Build history of the part. All positions in model axes, mm. A direction names the side the tool comes from. Round coordinates to 2 decimals unless told otherwise and drop trailing zeros. Write each loop counter-clockwise with the first axis right and the second up, starting at its lowest first coordinate (ties: lowest second). Pieces come first, ordered by that corner, then holes. Notation, with made-up numbers: M 61.5,-22 L 114.5,-22 A18 cw 114.5,5 Z; hole C 52,54.25 d9. An arc over 180 degrees is marked long. Use a Markdown table: item, result.
from build123d import *

# Parameters (mm, degrees)
TOP_ENVELOPE_START         = 8
CASEENVELOPE_W             = 92
CASEENVELOPE_H             = 63
TOP_ENVELOPE_DEPTH         = 17
OUTSIDE_R3_R               = 3
SHELL_1_T                  = -2
SIDEPORT_CLEARANCE_1_START = 6.45
SIDEPORT_PROFILE_1_W       = 10.1
SIDEPORT_PROFILE_1_H       = 13
SIDEPORT_CLEARANCE_1_DEPTH = 4.5
SIDEPORT_CLEARANCE_2_START = 6.45
SIDEPORT_PROFILE_2_W       = 7.7
SIDEPORT_PROFILE_2_H       = 13
SIDEPORT_CLEARANCE_2_DEPTH = 4.7
SIDEPORT_CLEARANCE_3_START = 6.45
SIDEPORT_PROFILE_3_W       = 7.7
SIDEPORT_PROFILE_3_H       = 13
SIDEPORT_CLEARANCE_3_DEPTH = 4.7
ENDPORT_CLEARANCE_1_START  = 6.45
ENDPORT_PROFILE_1_W        = 11
ENDPORT_PROFILE_1_H        = 17.3
ENDPORT_CLEARANCE_1_DEPTH  = 14.6
ENDPORT_CLEARANCE_2_START  = 6.45
ENDPORT_PROFILE_2_W        = 11
ENDPORT_PROFILE_2_H        = 14.7
ENDPORT_CLEARANCE_2_DEPTH  = 16.3
ENDPORT_CLEARANCE_3_START  = 6.45
ENDPORT_PROFILE_3_W        = 11
ENDPORT_PROFILE_3_H        = 14.7
ENDPORT_CLEARANCE_3_DEPTH  = 16.3
COOLING_SLOTS_START        = 22.5
COOLING_SLOTS_DEPTH        = 3


with BuildPart() as part:
    # CaseEnvelope → Top_Envelope (new body)
    with BuildSketch(Plane.XY.offset(TOP_ENVELOPE_START)):
        Rectangle(CASEENVELOPE_W, CASEENVELOPE_H)
    extrude(amount=TOP_ENVELOPE_DEPTH)

    # Outside_R3
    outside_r3_edges = [part.edges().sort_by_distance(p)[0] for p in [
        (46, -31.5, 16.5),
        (-46, -31.5, 16.5),
        (-46, 31.5, 16.5),
        (46, 31.5, 16.5),
    ]]
    fillet(outside_r3_edges, radius=OUTSIDE_R3_R)

    # Shell 1
    shell_1_openings = [part.faces().sort_by_distance(p)[0] for p in [
        (0, 0, 8),
    ]]
    offset(amount=SHELL_1_T, openings=shell_1_openings, kind=Kind.INTERSECTION)

    # SidePort_Profile_1 → SidePort_Clearance_1 (cut)
    with BuildSketch(Plane.XY.offset(SIDEPORT_CLEARANCE_1_START)):
        with Locations((-31.3, -33.5)):
            Rectangle(SIDEPORT_PROFILE_1_W, SIDEPORT_PROFILE_1_H)
    extrude(amount=SIDEPORT_CLEARANCE_1_DEPTH, mode=Mode.SUBTRACT)

    # SidePort_Profile_2 → SidePort_Clearance_2 (cut)
    with BuildSketch(Plane.XY.offset(SIDEPORT_CLEARANCE_2_START)):
        with Locations((-16.7, -33.5)):
            Rectangle(SIDEPORT_PROFILE_2_W, SIDEPORT_PROFILE_2_H)
    extrude(amount=SIDEPORT_CLEARANCE_2_DEPTH, mode=Mode.SUBTRACT)

    # SidePort_Profile_3 → SidePort_Clearance_3 (cut)
    with BuildSketch(Plane.XY.offset(SIDEPORT_CLEARANCE_3_START)):
        with Locations((-3.3, -33.5)):
            Rectangle(SIDEPORT_PROFILE_3_W, SIDEPORT_PROFILE_3_H)
    extrude(amount=SIDEPORT_CLEARANCE_3_DEPTH, mode=Mode.SUBTRACT)

    # EndPort_Profile_1 → EndPort_Clearance_1 (cut)
    with BuildSketch(Plane.XY.offset(ENDPORT_CLEARANCE_1_START)):
        with Locations((47.5, -17.8)):
            Rectangle(ENDPORT_PROFILE_1_W, ENDPORT_PROFILE_1_H)
    extrude(amount=ENDPORT_CLEARANCE_1_DEPTH, mode=Mode.SUBTRACT)

    # EndPort_Profile_2 → EndPort_Clearance_2 (cut)
    with BuildSketch(Plane.XY.offset(ENDPORT_CLEARANCE_2_START)):
        with Locations((47.5, 1.1)):
            Rectangle(ENDPORT_PROFILE_2_W, ENDPORT_PROFILE_2_H)
    extrude(amount=ENDPORT_CLEARANCE_2_DEPTH, mode=Mode.SUBTRACT)

    # EndPort_Profile_3 → EndPort_Clearance_3 (cut)
    with BuildSketch(Plane.XY.offset(ENDPORT_CLEARANCE_3_START)):
        with Locations((47.5, 19)):
            Rectangle(ENDPORT_PROFILE_3_W, ENDPORT_PROFILE_3_H)
    extrude(amount=ENDPORT_CLEARANCE_3_DEPTH, mode=Mode.SUBTRACT)

    # Cooling_Slot_Profiles → Cooling_Slots (cut)
    with BuildSketch(Plane.XY.offset(COOLING_SLOTS_START)):
        with BuildLine():
            Line((-23.81, -17.4), (18.81, -17.4))
            ThreePointArc((18.81, -17.4), (19.65145707, -17.05145707), (20, -16.21))
            Line((20, -16.21), (20, -16.19))
            ThreePointArc((20, -16.19), (19.65145707, -15.34854293), (18.81, -15))
            Line((18.81, -15), (-23.81, -15))
            ThreePointArc((-23.81, -15), (-24.65145707, -15.34854293), (-25, -16.19))
            Line((-25, -16.19), (-25, -16.21))
            ThreePointArc((-25, -16.21), (-24.65145707, -17.05145707), (-23.81, -17.4))
        make_face()
        with BuildLine():
            Line((-23.81, -12), (18.81, -12))
            ThreePointArc((18.81, -12), (19.65145707, -11.65145707), (20, -10.81))
            Line((20, -10.81), (20, -10.79))
            ThreePointArc((20, -10.79), (19.65145707, -9.94854293), (18.81, -9.6))
            Line((18.81, -9.6), (-23.81, -9.6))
            ThreePointArc((-23.81, -9.6), (-24.65145707, -9.94854293), (-25, -10.79))
            Line((-25, -10.79), (-25, -10.81))
            ThreePointArc((-25, -10.81), (-24.65145707, -11.65145707), (-23.81, -12))
        make_face()
        with BuildLine():
            Line((-23.81, -6.6), (18.81, -6.6))
            ThreePointArc((18.81, -6.6), (19.65145707, -6.25145707), (20, -5.41))
            Line((20, -5.41), (20, -5.39))
            ThreePointArc((20, -5.39), (19.65145707, -4.54854293), (18.81, -4.2))
            Line((18.81, -4.2), (-23.81, -4.2))
            ThreePointArc((-23.81, -4.2), (-24.65145707, -4.54854293), (-25, -5.39))
            Line((-25, -5.39), (-25, -5.41))
            ThreePointArc((-25, -5.41), (-24.65145707, -6.25145707), (-23.81, -6.6))
        make_face()
        with BuildLine():
            Line((-23.81, -1.2), (18.81, -1.2))
            ThreePointArc((18.81, -1.2), (19.65145707, -0.85145707), (20, -0.01))
            Line((20, -0.01), (20, 0.01))
            ThreePointArc((20, 0.01), (19.65145707, 0.85145707), (18.81, 1.2))
            Line((18.81, 1.2), (-23.81, 1.2))
            ThreePointArc((-23.81, 1.2), (-24.65145707, 0.85145707), (-25, 0.01))
            Line((-25, 0.01), (-25, -0.01))
            ThreePointArc((-25, -0.01), (-24.65145707, -0.85145707), (-23.81, -1.2))
        make_face()
        with BuildLine():
            Line((-23.81, 4.2), (18.81, 4.2))
            ThreePointArc((18.81, 4.2), (19.65145707, 4.54854293), (20, 5.39))
            Line((20, 5.39), (20, 5.41))
            ThreePointArc((20, 5.41), (19.65145707, 6.25145707), (18.81, 6.6))
            Line((18.81, 6.6), (-23.81, 6.6))
            ThreePointArc((-23.81, 6.6), (-24.65145707, 6.25145707), (-25, 5.41))
            Line((-25, 5.41), (-25, 5.39))
            ThreePointArc((-25, 5.39), (-24.65145707, 4.54854293), (-23.81, 4.2))
        make_face()
        with BuildLine():
            Line((-23.81, 9.6), (18.81, 9.6))
            ThreePointArc((18.81, 9.6), (19.65145707, 9.94854293), (20, 10.79))
            Line((20, 10.79), (20, 10.81))
            ThreePointArc((20, 10.81), (19.65145707, 11.65145707), (18.81, 12))
            Line((18.81, 12), (-23.81, 12))
            ThreePointArc((-23.81, 12), (-24.65145707, 11.65145707), (-25, 10.81))
            Line((-25, 10.81), (-25, 10.79))
            ThreePointArc((-25, 10.79), (-24.65145707, 9.94854293), (-23.81, 9.6))
        make_face()
        with BuildLine():
            Line((-23.81, 15), (18.81, 15))
            ThreePointArc((18.81, 15), (19.65145707, 15.34854293), (20, 16.19))
            Line((20, 16.19), (20, 16.21))
            ThreePointArc((20, 16.21), (19.65145707, 17.05145707), (18.81, 17.4))
            Line((18.81, 17.4), (-23.81, 17.4))
            ThreePointArc((-23.81, 17.4), (-24.65145707, 17.05145707), (-25, 16.21))
            Line((-25, 16.21), (-25, 16.19))
            ThreePointArc((-25, 16.19), (-24.65145707, 15.34854293), (-23.81, 15))
        make_face()
    extrude(amount=COOLING_SLOTS_DEPTH, mode=Mode.SUBTRACT)


solid = part.part
Q1. Drop flat-ended pins along their axis: P1, Ø1.6, axis at y = -30.5, z = 9, coming from the -X side; P2, Ø1.6, axis at x = -16, y = -30.5, coming from the -Z side; P3, Ø1, axis at y = -30, z = 9, coming from the +X side. Give the stop position or say it passes through.
Response values:
| item | result |
|---|---|
| P1 | stops at x = -45.75 |
| P2 | stops at z = 11.15 |
| P3 | stops at x = 45.83 |
Q2. Cut at A-A on z = 18.25. Give the cut face in (x, y), and give its area (3 significant figures).
Response values:
| item | result |
|---|---|
| outline | M -46,-28.5 A3 ccw -43,-31.5 L 43,-31.5 A3 ccw 46,-28.5 L 46,-26.45 L 44,-26.45 L 44,-28.5 A1 cw 43,-29.5 L -43,-29.5 A1 cw -44,-28.5 L -44,28.5 A1 cw -43,29.5 L 43,29.5 A1 cw 44,28.5 L 44,26.35 L 46,26.35 L 46,28.5 A3 ccw 43,31.5 L -43,31.5 A3 ccw -46,28.5 Z; M 44,-9.15 L 46,-9.15 L 46,-6.25 L 44,-6.25 Z; M 44,8.45 L 46,8.45 L 46,11.65 L 44,11.65 Z |
| area | 504 mm2 |
Q3. Cut at B-B on y = -13.5. Give the cut face in (x, z).
Response values:
| item | result |
|---|---|
| outline | M -46,8 L -44,8 L -44,23 L 44,23 L 44,21.05 L 46,21.05 L 46,25 L -46,25 Z |
Q4. Which spindle directions (+Z, -Z, +X, -X, +Y, -Y) get a long thin tool onto all of the face, cutting with end or side? Do faces 1 (the flat face through (-3, -1.2, 24)), 2 (the flat face through (-36.35, -31, 9)), 3 (the flat face through (45, 19, 22.75)), 4 (the cylindrical face through (45.1, -30.64, 16.62)), 5 (the flat face through (-1, 31.5, 16)). Say none if no direction does.
Response values:
| item | result |
|---|---|
| face 1 | +Z, -Z |
| face 2 | -Z, -Y |
| face 3 | -Z, +X |
| face 4 | +Z, -Z, +X, -Y |
| face 5 | +Z, -Z, +X, -X, +Y |
Q5. Two-plate mould, pull along Y, no slides. Class faces 6 (the flat face through (-2, -15, 24)), 7 (the cylindrical face through (-45.14, 30.6, 16.62)), 8 (the flat face through (45, 8.45, 15)), 9 (the flat face through (-7.15, -31, 10)): +Y half, -Y half, draft (parallel to the pull), parting line (faces both ways), or undercut.
Response values:
| item | result |
|---|---|
| face 6 | undercut |
| face 7 | +Y half |
| face 8 | undercut |
| face 9 | draft |
Q6. Drill centre lines: L1, parallel to Y at x = -29, z = 14; L2, parallel to X at y = 28.5, z = 19.75; L3, parallel to Z at x = 23, y = 0. Where is each one in solid material? Low to high.
Response values:
| item | result |
|---|---|
| L1 | y = -31.5 to -29.5, 29.5 to 31.5 |
| L2 | x = -46 to -44, 44 to 46 |
| L3 | z = 23 to 25 |
Q7. Cut at C-C on x = -17. Count the separate pieces of the cut face and the enclosed holes in it, and give its area (3 significant figures).
Response values:
| item | result |
|---|---|
| separate pieces | 8 |
| enclosed holes | 0 |
| area | 146 mm2 |
